Check sheet for the modelled part. Datum: model origin and axes. Units: mm. Round coordinates to 2 decimals unless told otherwise and drop trailing zeros. Order: outer loops, then holes, each group sorted by start corner. A loop starts at its lowest first (then second) coordinate and runs counter-clockwise, first axis right, second up.
Q1. Cross-section at A-A on x = 14.75. Record the cut outline in (y, z) (3 decimals).
Q2. Depth check by flat-ended pin: P1, Ø1, axis at x = 13.5, z = -12, coming from the +Y side. Enter the tip coordinate at first touch or a pass-through.
Q3. Mould release check, pull along Z, two halves, no side actions. Record for faces 1 (the flat face through (9, 0, -8)), 2 (the flat face through (9.022, 3.993, -1.516)), 3 (the cylindrical face through (0.07, 4.64, -7.48)), 4 (the flat face through (9, 2, -15.875)): +Z half, -Z half, draft (parallel to the pull), parting line (faces both ways), or undercut.
Q4. Scan lines: probe 1 along Z at (x, y) = (11.25, 4.1) (3 decimals); probe 2 along X at (y, z) = (4.55, -8); probe 3 along Y at (x, z) = (10.5, -8.5). Record each from-to range of solid material in increasing order.
from build123d import *

# Parameters (mm, degrees)
BOSS_EXTRUDE1_DEPTH = 18.25625
FILLET1_R           = 0.635
FILLET2_R           = 0.254
SKETCH2_W           = 15.20825
SKETCH2_H           = 1.528516132
CUT_EXTRUDE1_DEPTH  = 0.127


with BuildPart() as part:
    # Sketch1 → Boss-Extrude1 (new body)
    with BuildSketch(Plane(origin=(0, 0, 0), x_dir=(0, 0, -1), z_dir=(1, 0, 0))):
        Polygon((0, 0), (15.875, 0), (15.875, 5.55625), (0, 3.96875), align=None)
    extrude(amount=BOSS_EXTRUDE1_DEPTH)

    # Fillet1
    fillet1_edges = [part.edges().sort_by_distance(p)[0] for p in [
        (9.128125, 5.55625, -15.875),
    ]]
    fillet(fillet1_edges, radius=FILLET1_R)

    # Fillet2
    fillet2_edges = [part.edges().sort_by_distance(p)[0] for p in [
        (18.25625, 2.427291449, -15.875),
        (0, 4.727590757, -7.588407569),
        (18.25625, 4.727590757, -7.588407569),
        (0, 5.325405257, -15.666088379),
        (18.25625, 5.325405257, -15.666088379),
        (0, 2.427291449, -15.875),
        (9.128125, 3.96875, 0),
    ]]
    fillet(fillet2_edges, radius=FILLET2_R)

    # Sketch2 → Cut-Extrude1 (cut)
    with BuildSketch(Plane(origin=(0, 3.929455446, 0.392945545), x_dir=(1, 0, 0), z_dir=(0, 0.99503719, 0.099503719))):
        with Locations((9.128125, 1.894772226)):
            Rectangle(SKETCH2_W, SKETCH2_H)
    extrude(amount=-CUT_EXTRUDE1_DEPTH, mode=Mode.SUBTRACT)


solid = part.part
Results found:
1. outline: (0, -15.875) - (4.855, -15.875) arc R0.635 ccw to (5.486, -15.177) - (4.194, -2.253) - (4.068, -2.266) - (3.916, -0.745) - (4.042, -0.732) - (3.992, -0.229) arc R0.254 ccw to (3.739, 0) - (0, 0) - close
2. P1: stops at y = 5.22
3. face 1: draft
3. face 2: undercut
3. face 3: +Z half
3. face 4: -Z half
4. probe 1: z = -15.875 to -2.262
4. probe 2: x = 0 to 18.25
4. probe 3: y = 0 to 4.82
